The model under review builds one solid part; all positions refer to its coordinate system, in mm. Face numbers are marked on the shaded views. A direction names the side the tool comes from. Round coordinates to 2 decimals unless told otherwise and drop trailing zeros. Loops run counter-clockwise (first coordinate to the right, second up) from the corner with the lowest first, then second, coordinate; pieces in that order, holes last. Notation, with made-up numbers: (22, 26) -> (81, 26) arc R22 cw to (81, 55) -> close; hole circle Ø4 at (69.25, 41.25). An arc over 180 degrees is marked (long way). Return JSON: item names as keys, results as strings. Group by question number.
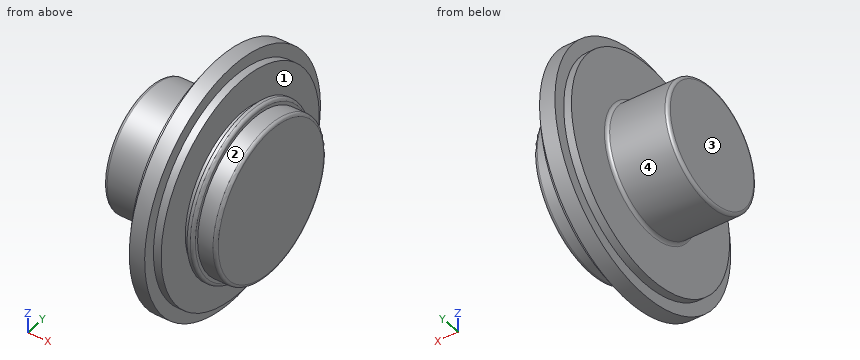
```python
from build123d import *

# Parameters (mm, degrees)
F2_R = 0.5


with BuildPart() as f1:
    # F0 (on Front) → F1 (revolve)
    with BuildSketch(Plane.XZ):
        Polygon((-20, 0), (0, 0), (0, 12.5), (-3, 12.5), (-3, 13.5), (-4, 13.5), (-4, 12.5), (-5, 12.5), (-5, 18), (-6.25, 18), (-6.25, 20), (-8.75, 20), (-8.75, 18), (-10, 18), (-10, 10), (-20, 10), align=None)
    revolve(axis=Axis((-10, 0, 0), (-1, 0, 0)))

    # F2
    f2_edges = [f1.edges().sort_by_distance(p)[0] for p in [
        (-10, 0, -10),
        (-20, 0, -10),
        (-15, 0, 10),
        (-3, 0, -13.5),
        (0, 0, -12.5),
    ]]
    fillet(f2_edges, radius=F2_R)


solid = f1.part
```
1. For P1, Ø1, axis at x = -7, z = -3.5, coming from the -Y side; P2, Ø2, axis at x = -7, y = 11, coming from the -Z side; P3, Ø18, axis at y = -5, z = 5, coming from the +X side; P4, Ø1.5, axis at y = -4.5, z = -15.5, coming from the +X side, all flat-tipped, find the tip position at first contact; note any pin that passes through.
2. We need section C-C, the plane x = -1.5. Write out the cut boundary in (y, z), then the cut area to 3 significant figures.
3. We need section B-B, the plane x = -12.5. Write out the cut boundary in (y, z), then the cut area to 3 significant figures.
4. Tool access review of the marked faces 1, 2, 3 and 4: name each direction out of +Z, -Z, +X, -X, +Y, -Y from which nothing blocks a thin tool from reaching the whole face with its end or side.
5. Wall thickness on line 1 (X direction, y = -4, z = 12); line 2 (X direction, y = -7.5, z = -14.5); line 3 (Y direction, x = -6.75, z = 16): over which ranges is each line inside the solid? List them lowest first.
6. We need section A-A, the plane y = -15.5. Write out the cut boundary in (x, z), then the cut area to 3 significant figures.
Check sheet entries:
{
 "1": {"P1": "stops at y = -19.77", "P2": "stops at z = -17.32", "P3": "stops at x = 0", "P4": "stops at x = -5"},
 "2": {"outline": "circle Ø25 at (0, 0)", "area": "491 mm²"},
 "3": {"outline": "circle Ø20 at (0, 0)", "area": "314 mm²"},
 "4": {"face 1": "none", "face 2": "+X", "face 3": "+Z, -Z, -X, +Y, -Y", "face 4": "-X"},
 "5": {"line 1": "x = -10 to -5, -4 to -3", "line 2": "x = -10 to -5", "line 3": "y = -12 to 12"},
 "6": {"outline": "(-10, -9.15) -> (-8.75, -9.15) -> (-8.75, -12.64) -> (-6.25, -12.64) -> (-6.25, -9.15) -> (-5, -9.15) -> (-5, 9.15) -> (-6.25, 9.15) -> (-6.25, 12.64) -> (-8.75, 12.64) -> (-8.75, 9.15) -> (-10, 9.15) -> close", "area": "109 mm²"}
}
